Read the model definition and answer for the solid it produces. Units are mm, in the model's axes. Face numbers are marked on the shaded views. A direction names the side the tool comes from. Give positions to 0.01 mm unless a question says otherwise; leave off trailing zeros. Write each loop counter-clockwise with the first axis right and the second up, starting at its lowest first coordinate (ties: lowest second). Pieces come first, ordered by that corner, then holes. Notation, with made-up numbers: (8, 68.5) -> (19, 68.5) arc R21 ccw to (19, 87.5) -> close; hole circle Ø7 at (53, -32). An arc over 180 degrees is marked (long way). Put each result on its own line as item: value. Start each with the question number.
from build123d import *

# Parameters (mm, degrees)
F2_R = 5.08


with BuildPart() as f1:
    # F0 (on Front) → F1 (revolve)
    with BuildSketch(Plane.XZ):
        Polygon((0, 7.581339), (0, 0), (67.31, 0), (67.31, 14.4018), (12.954, 14.4018), (12.954, 7.581339), align=None)
    revolve(axis=Axis((33.655, 0, 0), (-1, 0, 0)))

    # F2
    f2_edges = [f1.edges().sort_by_distance(p)[0] for p in [
        (67.31, 0, -14.4018),
        (12.954, 0, -14.4018),
        (40.132, 0, 14.4018),
        (0, 0, -7.581339),
    ]]
    fillet(f2_edges, radius=F2_R)


solid = f1.part
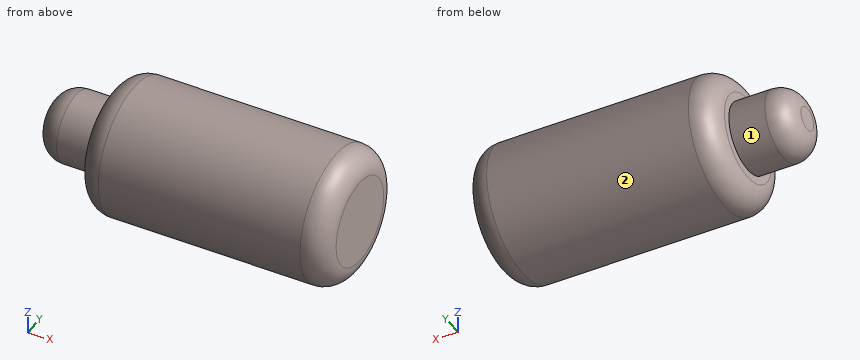
1) A cutting plane is placed at A-A on x = 30. Give the vertices of the cut face in (y, z), and give its area (3 significant figures).
2) Each of these flat-tipped pins is pushed along its axis until it touches: pin 1 Ø12 at (x, y) = (55.5, 6) entering from -Z; pin 2 Ø10 at (y, z) = (-3.5, 10) entering from -X; pin 3 Ø12 at (y, z) = (-7, 7.5) entering from -X; pin 4 Ø1.5 at (y, z) = (0.5, 11) entering from -X. Where does it stop, or does it pass through?
3) Straight lines are drawn through the part: line 1 (X direction, y = -5.75, z = 6.5); line 2 (Z direction, x = 21, y = -6.25); line 3 (Y direction, x = 24, z = -6). For each, find the intervals that lie inside material, in ascending order. Write a range as [from, to].
4) A cutting plane is placed at B-B on x = 8. Give the vertices of the cut face in (y, z), and give its area (3 significant figures).
5) For the marked faces 1 and 2, determine the directions among +Z, -Z, +X, -X, +Y, -Y from which every point of the face is accessible in a straight line to the end or side of a thin tool.
Results found:
1. outline: circle Ø28.8 at (0, 0)
1. area: 652 mm²
2. pin 1: stops at z = -14.4
2. pin 2: stops at x = 1.05
2. pin 3: stops at x = 0.31
2. pin 4: stops at x = 13.04
3. line 1: x = [12.95, 67.31]
3. line 2: z = [-12.97, 12.97]
3. line 3: y = [-13.09, 13.09]
4. outline: circle Ø15.16 at (0, 0)
4. area: 181 mm²
5. face 1: -X
5. face 2: +X, -X
